```python
from build123d import *

# Parameters (mm, degrees)
CROQUIS1_R              = 42.5
SALIENTE_EXTRUIR1_DEPTH = 30
CROQUIS2_R              = 2.5
CORTAR_EXTRUIR1_DEPTH   = 10
CROQUIS3_R              = 27.5
CORTAR_EXTRUIR2_DEPTH   = 5
CROQUIS4_R              = 2
CORTAR_EXTRUIR3_DEPTH   = 66.096082831


with BuildPart() as part:
    # Croquis1 → Saliente-Extruir1 (new body)
    with BuildSketch(Plane(origin=(0, 0, 0), x_dir=(1, 0, 0), z_dir=(0, 1, 0))):
        with Locations(Location((0, 0, 0), (0, 0, 270))):
            Circle(CROQUIS1_R)
    extrude(amount=SALIENTE_EXTRUIR1_DEPTH)

    # Croquis2 → Cortar-Extruir1 (cut)
    with BuildSketch(Plane(origin=(0, 30, 0), x_dir=(1, 0, 0), z_dir=(0, 1, 0))):
        with Locations(Location((0, 0, 0), (0, 0, 270))):
            Circle(CROQUIS2_R)
    extrude(amount=-CORTAR_EXTRUIR1_DEPTH, mode=Mode.SUBTRACT)

    # Croquis3 → Cortar-Extruir2 (cut)
    with BuildSketch(Plane.XZ):
        with Locations(Location((0, 0, 0), (0, 0, 270))):
            Circle(CROQUIS3_R)
    extrude(amount=-CORTAR_EXTRUIR2_DEPTH, mode=Mode.SUBTRACT)

    # Croquis4 → Cortar-Extruir3 (cut, through all)
    with BuildSketch(Plane.XZ.offset(-5)):
        with Locations(Location((0, 20, 0), (0, 0, 270))):
            Circle(CROQUIS4_R)
        with Locations(Location((-20, 0, 0), (0, 0, 270))):
            Circle(CROQUIS4_R)
        with Locations(Location((0, -20, 0), (0, 0, 270))):
            Circle(CROQUIS4_R)
        with Locations(Location((20, 0, 0), (0, 0, 270))):
            Circle(CROQUIS4_R)
    extrude(amount=-CORTAR_EXTRUIR3_DEPTH, mode=Mode.SUBTRACT)


solid = part.part
```
Input: part model. Units: mm. Frame: model coordinates. A direction names the side the tool comes from. Coordinates: 2 decimals unless noted, no trailing zeros. Write each loop counter-clockwise with the first axis right and the second up, starting at its lowest first coordinate (ties: lowest second). Pieces come first, ordered by that corner, then holes.
1) Section B-B on x = 21. Output: boundary loops of the cut face in (y, z), and give its area (3 significant figures).
2) Pin query (flat end, axial travel): pin 1 Ø1.5 at (x, y) = (-20, 6.5) entering from -Z; pin 2 Ø6 at (x, z) = (10, -21.5) entering from -Y; pin 3 Ø3 at (y, z) = (20.5, 23.5) entering from +X. Return the tip coordinate at first contact, or that it passes through.
3) Section D-D on z = -20. Output: boundary loops of the cut face in (x, y), and give its area (3 significant figures).
4) Mould query, pull axis Z, two halves, no side actions, for faces 4 (the cylindrical face through (-2.44, 25.07, -0.54)), 5 (the flat face through (-9, 30, -1)), 6 (the cylindrical face through (-25.861, 14.79, -33.727)). Classes: pulls with the +Z half, pulls with the -Z half, needs draft (parallel to the pull), parting line crosses it, or undercut.
5) Section A-A on x = 0. Output: boundary loops of the cut face in (y, z).
6) Material intervals for line 1 along X through (y, z) = (21.5, 0); line 2 along X through (y, z) = (16.5, 0); line 3 along Z through (x, y) = (-1, 12.75), sorted ascending.
7) Set-up query: faces 1 (the cylindrical face through (-18, 17, 0)), 2 (the flat face through (0, 5, 0)), 3 (the flat face through (0, 20, 0)). Return all of +Z, -Z, +X, -X, +Y, -Y with unobstructed straight access to the full face (end or side cutting, diameter ignored); none if empty.
8) Section C-C on y = 14.25. Output: boundary loops of the cut face in (x, z), and give its area (3 significant figures).
Check result:
1. outline: (0, -36.95) - (30, -36.95) - (30, -1.73) - (5, -1.73) - (5, -17.76) - (0, -17.76) - close; (0, 17.76) - (5, 17.76) - (5, 1.73) - (30, 1.73) - (30, 36.95) - (0, 36.95) - close
1. area: 1,950 mm2
2. pin 1: stops at z = -37.89
2. pin 2: stops at y = 5
2. pin 3: stops at x = 36.36
3. outline: (-37.5, 0) - (-18.87, 0) - (-18.87, 5) - (-2, 5) - (-2, 30) - (-37.5, 30) - close; (2, 5) - (18.87, 5) - (18.87, 0) - (37.5, 0) - (37.5, 30) - (2, 30) - close
3. area: 1,960 mm2
4. face 4: undercut
4. face 5: needs draft
4. face 6: parting line crosses it
5. outline: (0, -42.5) - (30, -42.5) - (30, -22) - (5, -22) - (5, -27.5) - (0, -27.5) - close; (0, 27.5) - (5, 27.5) - (5, 22) - (30, 22) - (30, 42.5) - (0, 42.5) - close; (5, -18) - (30, -18) - (30, -2.5) - (20, -2.5) - (20, 2.5) - (30, 2.5) - (30, 18) - (5, 18) - close
6. line 1: x = -42.5 to -22, -18 to -2.5, 2.5 to 18, 22 to 42.5
6. line 2: x = -42.5 to -22, -18 to 18, 22 to 42.5
6. line 3: z = -42.49 to -21.73, -18.27 to 18.27, 21.73 to 42.49
7. face 1: +Y, -Y
7. face 2: -Y
7. face 3: +Y
8. outline: circle Ø85 at (0, 0); hole circle Ø4 at (-20, 0); hole circle Ø4 at (0, -20); hole circle Ø4 at (0, 20); hole circle Ø4 at (20, 0)
8. area: 5,620 mm2
